Could you check a few things on this model? Use its own coordinates, in mm. A direction names the side the tool comes from. Coordinates: 2 decimals unless noted, no trailing zeros. Write each loop counter-clockwise with the first axis right and the second up, starting at its lowest first coordinate (ties: lowest second). Pieces come first, ordered by that corner, then holes.
Item 1: Which directions (+Z, -Z, +X, -X, +Y, -Y) give clear straight access to the entire face, cutting with the end or side of a thin tool? Please do faces 1 (the cylindrical face through (41, 0, 15)), 2 (the flat face through (-10, -5, 10)).
Item 2: I want a section at C-C on z = 13. Please give me the cut outline in (x, y), then the cut area to 3 significant figures.
Item 3: I want a section at B-B on z = 6.5. Please give me the cut outline in (x, y), then the cut area to 3 significant figures.
Item 4: For P1, Ø3, axis at x = 0, y = 0, coming from the -Z side; P2, Ø1.2, axis at x = 18, z = 3, coming from the +Y side; P3, Ø6, axis at y = -2, z = 21.5, coming from the +X side; P4, Ø3, axis at x = -8.5, y = 1.5, coming from the +Z side, each with a flat end and sliding along its axis, tell me the tip position at first contact or that it passes through.
Item 5: Thinking about a two-plate mould opening in X: for faces 3 (the flat face through (-21.65, 0, 13)), 4 (the flat face through (32.3, -1.3, 26)), 5 (the cylindrical face through (52.5, 0.07, 8.07)), 6 (the cylindrical face through (29.35, -0.07, 12.82)), which applies, +X half, -X half, draft (parallel to the pull), parting line (faces both ways), or undercut?
Item 6: I want a section at A-A on x = -14.5. Please give me the cut outline in (y, z), then the cut area to 4 significant figures.
Item 7: If I drill on probe 1 along X at (y, z) = (-2.75, 13); probe 2 along X at (y, z) = (1.25, 2.5); probe 3 along Z at (x, y) = (12, -1), over which ranges is the centre line in solid material (lowest first)?
Item 8: I want a section at D-D on y = 0. State how many separate pieces and enclosed holes the cut face has, then the cut area to 3 significant figures.
Autodesk Inventor part; units mm, degrees
ref_plane "YZ Plane" through (0, 0, 0) normal (1, 0, 0) x (0, 1, 0)
ref_plane "XZ Plane" through (0, 0, 0) normal (0, 1, 0) x (-1, 0, 0)
ref_plane "XY Plane" through (0, 0, 0) normal (0, 0, 1) x (1, 0, 0)
sketch "Sketch1" plane through (0, 0, 0) normal (0, 0, 1) x (1, 0, 0)
  circle A0 centre (0, 0) radius 1.65
  circle A1 centre (0, 0) radius 3
  circle A2 centre (31, 0) radius 1.65
  circle A3 centre (31, 0) radius 3
  dimension "d0" = 3.3
  dimension "d1" = 6
  dimension "d22" = 31
extrude "Extrusion1" add sketch "Sketch1" along normal blind 26
sketch "Sketch2" plane through (0, 0, 0) normal (0, 0, -1) x (-1, 0, 0)
  circle A0 centre (0, 0) radius 3
  circle A1 centre (0, 0) radius 5
  circle A2 centre (-31, 0) radius 1.65
  circle A3 centre (-31, 0) radius 5
  circle A4 centre (0, 0) radius 1.65 construction
  line L0 (-29.35, 2) -> (-1.65, 2)
  line L1 (-1.65, 2) -> (-1.65, -2)
  line L2 (-1.65, -2) -> (-29.35, -2)
  line L3 (-29.35, -2) -> (-29.35, 2)
  point P0 (-1.65, 0)
  dimension "d4" = 10
  dimension "d7" = 4
extrude "Extrusion2" add sketch "Sketch2" against normal blind 4 contours A0 L0 A1 L2 | L0 L1 L2 A0 | A0 L2 A1 L0 | A1 L2 A3 L0 | L0 L3 L2 A3 | A3 L2 L3 L0 picked at (-2.1, 0)
sketch "Sketch3" plane through (0, 0, 0) normal (0, 0, -1) x (-1, 0, 0)
  line L0 (-52.65, -5) -> (-32.65, -5)
  line L1 (-32.65, -5) -> (-32.65, 5)
  line L2 (-32.65, 5) -> (-52.65, 5)
  line L3 (-52.65, 5) -> (-52.65, -5)
  line L4 (1.65, 5) -> (21.65, 5)
  line L5 (21.65, 5) -> (21.65, -5)
  line L6 (21.65, -5) -> (1.65, -5)
  line L7 (1.65, -5) -> (1.65, 5)
  circle A0 centre (0, 0) radius 1.65 construction
  circle A1 centre (-31, 0) radius 1.65 construction
  arc A2 (-26.4174, 2) -> (-26.4174, -2) centre (-31, 0) ccw construction
  arc A3 (-4.5826, -2) -> (-4.5826, 2) centre (0, 0) ccw construction
  point P0 (-32.65, 0)
  point P1 (1.65, 0)
  dimension "d8" = 20
  dimension "d10" = 20
extrude "Extrusion3" add sketch "Sketch3" against normal blind 20
sketch "Sketch4" plane through (32.65, 5, 0) normal (0, 1, 0) x (1, 0, 0)
  circle A0 centre (-47.15, -13) radius 4
  circle A1 centre (12.85, -13) radius 4
  line L0 (-34.3, -20) -> (-54.3, -20)
  line L1 (20, -20) -> (0, -20)
  line L2 (-34.3, 0) -> (-54.3, 0)
  line L3 (20, 0) -> (20, -20)
  line L4 (-54.3, 0) -> (-54.3, -20)
  point P0 (-32.65, 0)
  point P1 (-44.3, -20)
  point P2 (10, -20)
  dimension "d13" = 8
  dimension "d14" = 8
  dimension "d15" = 13
  dimension "d23" = 60
  dimension "d24" = 7.15
  dimension "d25" = 7.15
extrude "Extrusion4" cut sketch "Sketch4" against normal blind 20
chamfer "Chamfer1" distance 8 angle 45 2 edges at (52.65, 0, 0) (-21.65, 0, 0)
fillet "Fillet1" radius 2 12 edges at (32.65, 2.5055, 12) (32.65, -2.5055, 12) (32.65, 5, 10) (-1.65, 2.5055, 12) (-1.65, -2.5055, 12) (-1.65, 5, 10) (-1.65, -5, 10) (32.65, -5, 10) (52.65, 0, 20) (52.65, 0, 8) (-21.65, 0, 8) (-21.65, 0, 20)
sketch "Sketch5" plane through (0, 0, 20) normal (0, 0, 1) x (1, 0, 0)
  line L0 (-19.65, -5) -> (-19.65, 5)
  arc A0 (0.21, 2.9926) -> (0.21, -2.9926) centre (0, 0) ccw
  circle A1 centre (-9, 0) radius 1
  circle A2 centre (40, 0) radius 1
  arc A3 (30.79, -2.9926) -> (30.79, 2.9926) centre (31, 0) ccw
  point P0 (-19.65, 0)
  dimension "d26" = 2
  dimension "d27" = 2
  dimension "d28" = 5
  dimension "d29" = 5
extrude "Extrusion5" cut sketch "Sketch5" against normal blind 10
equation "\"d10\" = d8"
equation "\"d24\" = d25"
equation "\"d29\" = d28"
properties part number "spacer stepperM n rail"
Response values:
1. face 1: +Z
1. face 2: +Z, -Z, +X, -X, -Y
2. outline: (-21.65, -5) - (-18.5, -5) - (-18.5, 5) - (-21.65, 5) - close; (-10.5, -5) - (-3.12, -5) arc R2 ccw to (-1.39, -3.99) arc R2 cw to (0.21, -2.99) arc R3 ccw to (0.21, 2.99) arc R2 cw to (-1.39, 3.99) arc R2 ccw to (-3.12, 5) - (-10.5, 5) - close; (30.79, -2.99) arc R2 cw to (32.39, -3.99) arc R2 ccw to (34.12, -5) - (41.5, -5) - (41.5, 5) - (34.12, 5) arc R2 ccw to (32.39, 3.99) arc R2 cw to (30.79, 2.99) arc R3 ccw to start; (49.5, -5) - (52.65, -5) - (52.65, 5) - (49.5, 5) - close; hole circle Ø2 at (-9, 0); hole circle Ø3.3 at (0, 0); hole circle Ø3.3 at (31, 0); hole circle Ø2 at (40, 0)
2. area: 267 mm2
3. outline: (-20.15, -5) - (-3.12, -5) arc R2 ccw to (-1.39, -3.99) arc R2 cw to (0.21, -2.99) arc R3 ccw to (0.21, 2.99) arc R2 cw to (-1.39, 3.99) arc R2 ccw to (-3.12, 5) - (-20.15, 5) - close; (30.79, -2.99) arc R2 cw to (32.39, -3.99) arc R2 ccw to (34.12, -5) - (51.15, -5) - (51.15, 5) - (34.12, 5) arc R2 ccw to (32.39, 3.99) arc R2 cw to (30.79, 2.99) arc R3 ccw to start; hole circle Ø3.3 at (0, 0); hole circle Ø3.3 at (31, 0)
3. area: 403 mm2
4. P1: passes through
4. P2: stops at y = 2
4. P3: stops at x = 52.59
4. P4: stops at z = 20
5. face 3: -X half
5. face 4: draft
5. face 5: +X half
5. face 6: undercut
6. outline: (-5, 0.85) - (5, 0.85) - (5, 9) - (-5, 9) - close; (-5, 17) - (5, 17) - (5, 20) - (-5, 20) - close
6. area: 111.5 mm2
7. probe 1: x = -21.65 to -18.5, -10.5 to 1.2, 29.8 to 41.5, 49.5 to 52.65
7. probe 2: x = -16.15 to -1.08, 1.08 to 29.92, 32.08 to 47.15
7. probe 3: z = 0 to 4
8. separate pieces: 3
8. enclosed holes: 2
8. area: 780 mm2
